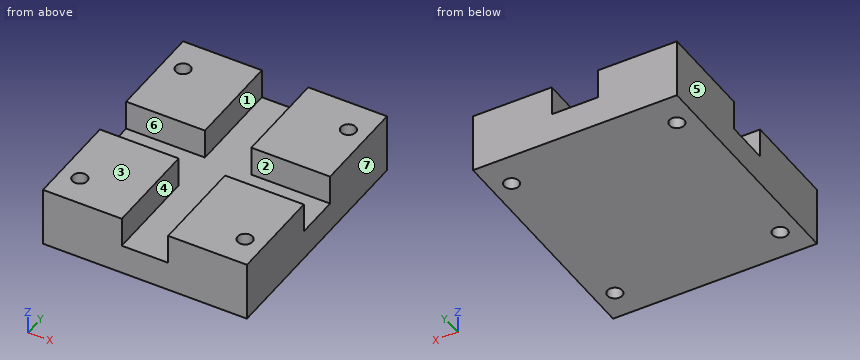
from build123d import *

# Parameters (mm, degrees)
F0_W     = 87.122
F0_H     = 101.6
F1_DEPTH = 12.7
F2_W     = 33.655
F2_H     = 41.275
F3_DEPTH = 12.7
F4_R     = 3.175
F5_DEPTH = 25.4


with BuildPart() as f1:
    # F0 (on Top) → F1 (new body)
    with BuildSketch(Plane.XY):
        with Locations((43.561, 50.8)):
            Rectangle(F0_W, F0_H)
    extrude(amount=F1_DEPTH)

    # F2 (on face) → F3 (join)
    with BuildSketch(Plane.XY.offset(12.7)):
        with Locations((16.8275, 80.9625)):
            Rectangle(F2_W, F2_H)
        with Locations((70.2945, 80.9625)):
            Rectangle(F2_W, F2_H)
        Polygon((53.467, 0), (87.122, 0), (87.122, 41.275), (77.888655, 41.275), (73.54703, 41.275), (53.467, 41.275), align=None)
        with Locations((16.8275, 20.6375)):
            Rectangle(F2_W, F2_H)
    extrude(amount=F3_DEPTH)

    # F4 (on face) → F5 (cut)
    with BuildSketch(Plane.XY.offset(25.4)):
        with Locations((78.867, 87.63)):
            Circle(F4_R)
        with Locations((8.255, 87.63)):
            Circle(F4_R)
        with Locations((78.867, 12.7)):
            Circle(F4_R)
        with Locations((8.255, 12.7)):
            Circle(F4_R)
    extrude(amount=-F5_DEPTH, mode=Mode.SUBTRACT)


solid = f1.part
Build history of the part. All positions in model axes, mm. Face numbers are marked on the shaded views. A direction names the side the tool comes from. Give positions to 0.01 mm unless a question says otherwise; leave off trailing zeros. Order: outer loops, then holes, each group sorted by start corner. A loop starts at its lowest first (then second) coordinate and runs counter-clockwise, first axis right, second up. Notation, with made-up numbers: M -4.5,-22.75 L 43.5,-22.75 A18 cw 43.5,5.25 Z; hole C 72.5,41.25 d7. An arc over 180 degrees is marked long. Put each result on its own line as item: value.
Item 1: Cut at D-D on y = 93. Write the cut outline in (x, z) (3 decimals).
Results are:
outline: M 0,0 L 87.122,0 L 87.122,25.4 L 53.467,25.4 L 53.467,12.7 L 33.655,12.7 L 33.655,25.4 L 0,25.4 Z
Item 2: Which spindle directions (+Z, -Z, +X, -X, +Y, -Y) get a long thin tool onto all of the face, cutting with end or side? Do the marked faces 1, 2 and 3. Say none if no direction does.
Results are:
face 1: +Z, +Y, -Y
face 2: +Z, +X, -X
face 3: +Z, +X, -X, +Y, -Y
Item 3: Pull direction X, two halves, no side cores. Call the marked faces 4, 5, 6 and 7: +X half, -X half, draft (parallel to the pull), parting line (faces both ways), or undercut.
Results are:
face 4: undercut
face 5: -X half
face 6: draft
face 7: +X half
Item 4: Wall check: probe 1 along Y at (x, z) = (81.5, 2); probe 2 along X at (y, z) = (93.5, 17) (3 decimals); probe 3 along Y at (x, z) = (8.5, 15.5) (3 decimals). Give the ranges that are in metal, low to high.
Results are:
probe 1: 0 to 10.93, 14.47 to 85.86, 89.4 to 101.6
probe 2: 0 to 33.655, 53.467 to 87.122
probe 3: 0 to 9.534, 15.866 to 41.275, 60.325 to 84.464, 90.796 to 101.6
Item 5: Drop a flat-ended pin along its axis: pin 1 Ø5.5 at (x, y) = (78.867, 12.7) entering from +Z. Give the stop position or say it passes through.
Results are:
pin 1: through
Item 6: Cut at C-C on x = 80. Write the cut outline in (y, z) (3 decimals), then the cut area to 3 significant figures.
Results are:
outline: M 0,0 L 9.734,0 L 9.734,25.4 L 0,25.4 Z; M 15.666,0 L 84.664,0 L 84.664,25.4 L 60.325,25.4 L 60.325,12.7 L 41.275,12.7 L 41.275,25.4 L 15.666,25.4 Z; M 90.596,0 L 101.6,0 L 101.6,25.4 L 90.596,25.4 Z
area: 2,040 mm2
Item 7: Cut at A-A on z = 19. Write the cut outline in (x, y) (3 decimals).
Results are:
outline: M 0,0 L 33.655,0 L 33.655,41.275 L 0,41.275 Z; M 0,60.325 L 33.655,60.325 L 33.655,101.6 L 0,101.6 Z; M 53.467,0 L 87.122,0 L 87.122,41.275 L 53.467,41.275 Z; M 53.467,60.325 L 87.122,60.325 L 87.122,101.6 L 53.467,101.6 Z; hole C 8.255,12.7 d6.35; hole C 8.255,87.63 d6.35; hole C 78.867,12.7 d6.35; hole C 78.867,87.63 d6.35
Item 8: Cut at B-B on y = 12.7. Write the cut outline in (x, z) (3 decimals).
Results are:
outline: M 0,0 L 5.08,0 L 5.08,25.4 L 0,25.4 Z; M 11.43,0 L 75.692,0 L 75.692,25.4 L 53.467,25.4 L 53.467,12.7 L 33.655,12.7 L 33.655,25.4 L 11.43,25.4 Z; M 82.042,0 L 87.122,0 L 87.122,25.4 L 82.042,25.4 Z
